from build123d import *

# Parameters (mm, degrees)
EXTRUDE_1_DEPTH      = 2
EXTRUDE_2_DEPTH      = 29
EXTRUDE_2_DEPTH_BACK = 2
CUT_EXTRUDE_5_REACH  = 63.117
SKETCH_3_R           = 0.75
SKETCH_3_W           = 9
SKETCH_3_H           = 20.1
CUT_EXTRUDE_7_REACH  = 63.924
SKETCH_12_R          = 0.75
SKETCH_12_W          = 9
SKETCH_12_H          = 20.1
CUT_EXTRUDE_8_REACH  = 75.269
SKETCH_13_R          = 1
SKETCH_13_W          = 16
SKETCH_13_H          = 40.897450577
EXTRUDE_START        = 15
SKETCH_15_R          = 2
SKETCH_15_R_2        = 1
EXTRUDE_9_DEPTH      = 15
CUT_EXTRUDE_9_REACH  = 63.508
SKETCH_16_W          = 5
SKETCH_16_H          = 20
EXTRUDE_10_DEPTH     = 24.1
EXTRUDE_11_DEPTH     = 1.5
CUT_EXTRUDE_10_REACH = 75.269
SKETCH_20_W          = 30
SKETCH_20_H          = 1.5
EXTRUDE_12_DEPTH     = 15
SKETCH_21_W          = 16
SKETCH_21_H          = 2
EXTRUDE_13_DEPTH     = 2
SKETCH_22_W          = 1
SKETCH_22_H          = 8
SKETCH_22_W_2        = 1.757464375
SKETCH_22_H_2        = 1.5298575
EXTRUDE_14_DEPTH     = 13
CUT_EXTRUDE_11_REACH = 64.018
SKETCH_23_W          = 12.5
SKETCH_23_H          = 12.2


with BuildPart() as part:
    # 草圖1 → 填料-伸長1 (new body)
    with BuildSketch(Plane.XY):
        Polygon((-15, 0), (15, 0), (17.19885826, 0), (20.767570176, -12.346175865), (15, -14), (15, -64), (-15, -64), (-15, -14), (-20.767570176, -12.346175865), (-17.227361215, 0), align=None)
    extrude(amount=EXTRUDE_1_DEPTH)

    # 草圖2 → 填料-伸長2 (add, two sides: drawn at the far end of the back side and taken through both)
    with BuildSketch(Plane.XY.offset(2).offset(-EXTRUDE_2_DEPTH_BACK)):
        Polygon((-19.940658108, -9.462390777), (19.934511943, -9.464160254), (20.767570176, -12.346175865), (11.154953216, -15.102549423), (-11.154953216, -15.102549423), (-20.767570176, -12.346175865), align=None)
    extrude(amount=EXTRUDE_2_DEPTH + EXTRUDE_2_DEPTH_BACK)

    # 草圖3 → 除料-伸長5 (cut, up to next)
    with BuildSketch(Plane(origin=(3.55693642, -17.281245681, 0), x_dir=(0.9612616959383193, 0.2756373558169973, 0), z_dir=(-0.2756373558169973, 0.9612616959383194, 0)), mode=Mode.PRIVATE) as cut_extrude_5_sk1:
        with Locations((13.397816779, -5.2)):
            Circle(SKETCH_3_R)
    cut_extrude_5_tool1 = extrude(cut_extrude_5_sk1.sketch, amount=CUT_EXTRUDE_5_REACH, mode=Mode.PRIVATE) & part.part
    # 草圖3 → 除料-伸長5 (cut, up to next)
    with BuildSketch(Plane(origin=(3.55693642, -17.281245681, 0), x_dir=(0.9612616959383193, 0.2756373558169973, 0), z_dir=(-0.2756373558169973, 0.9612616959383194, 0)), mode=Mode.PRIVATE) as cut_extrude_5_sk2:
        with Locations((13.397816779, -28.7)):
            Circle(SKETCH_3_R)
    cut_extrude_5_tool2 = extrude(cut_extrude_5_sk2.sketch, amount=CUT_EXTRUDE_5_REACH, mode=Mode.PRIVATE) & part.part
    # 草圖3 → 除料-伸長5 (cut, up to next)
    with BuildSketch(Plane(origin=(3.55693642, -17.281245681, 0), x_dir=(0.9612616959383193, 0.2756373558169973, 0), z_dir=(-0.2756373558169973, 0.9612616959383194, 0)), mode=Mode.PRIVATE) as cut_extrude_5_sk3:
        with Locations((13.397816779, -16.95)):
            Rectangle(SKETCH_3_W, SKETCH_3_H)
    cut_extrude_5_tool3 = extrude(cut_extrude_5_sk3.sketch, amount=CUT_EXTRUDE_5_REACH, mode=Mode.PRIVATE) & part.part
    add(cut_extrude_5_tool1.solids().sort_by_distance((16.435744, -13.588307, 5.2))[0], mode=Mode.SUBTRACT)
    add(cut_extrude_5_tool2.solids().sort_by_distance((16.435744, -13.588307, 28.7))[0], mode=Mode.SUBTRACT)
    add(cut_extrude_5_tool3.solids().sort_by_distance((16.435744, -13.588307, 16.95))[0], mode=Mode.SUBTRACT)

    # 除料-伸長7: up to this plane
    cut_extrude_7_end = Plane(origin=(-19.940658108, -9.462390777, 0), z_dir=(4.437541139610382e-05, 0.9999999990154116, 0))
    # 草圖12 → 除料-伸長7 (cut, up to the surface)
    with BuildSketch(Plane(origin=(-4.849074128, -16.910731155, 0), x_dir=(0.9612616959383179, -0.2756373558170027, 0), z_dir=(-0.2756373558170027, -0.9612616959383179, 0)), mode=Mode.PRIVATE) as cut_extrude_7_sk1:
        with Locations((-12.060002458, 28.7)):
            Circle(SKETCH_12_R)
    cut_extrude_7_tool1 = split(extrude(cut_extrude_7_sk1.sketch, amount=-CUT_EXTRUDE_7_REACH, mode=Mode.PRIVATE), bisect_by=cut_extrude_7_end, keep=Keep.BOTH, mode=Mode.PRIVATE)
    add(cut_extrude_7_tool1.solids().sort_by_distance((-16.441893, -13.586544, 28.7))[0], mode=Mode.SUBTRACT)
    # 草圖12 → 除料-伸長7 (cut, up to the surface)
    with BuildSketch(Plane(origin=(-4.849074128, -16.910731155, 0), x_dir=(0.9612616959383179, -0.2756373558170027, 0), z_dir=(-0.2756373558170027, -0.9612616959383179, 0)), mode=Mode.PRIVATE) as cut_extrude_7_sk2:
        with Locations((-12.060002458, 5.2)):
            Circle(SKETCH_12_R)
    cut_extrude_7_tool2 = split(extrude(cut_extrude_7_sk2.sketch, amount=-CUT_EXTRUDE_7_REACH, mode=Mode.PRIVATE), bisect_by=cut_extrude_7_end, keep=Keep.BOTH, mode=Mode.PRIVATE)
    add(cut_extrude_7_tool2.solids().sort_by_distance((-16.441893, -13.586544, 5.2))[0], mode=Mode.SUBTRACT)
    # 草圖12 → 除料-伸長7 (cut, up to the surface)
    with BuildSketch(Plane(origin=(-4.849074128, -16.910731155, 0), x_dir=(0.9612616959383179, -0.2756373558170027, 0), z_dir=(-0.2756373558170027, -0.9612616959383179, 0)), mode=Mode.PRIVATE) as cut_extrude_7_sk3:
        with Locations((-12.060002458, 16.95)):
            Rectangle(SKETCH_12_W, SKETCH_12_H)
    cut_extrude_7_tool3 = split(extrude(cut_extrude_7_sk3.sketch, amount=-CUT_EXTRUDE_7_REACH, mode=Mode.PRIVATE), bisect_by=cut_extrude_7_end, keep=Keep.BOTH, mode=Mode.PRIVATE)
    add(cut_extrude_7_tool3.solids().sort_by_distance((-16.441893, -13.586544, 16.95))[0], mode=Mode.SUBTRACT)

    # 草圖13 → 除料-伸長8 (cut, up to next)
    with BuildSketch(Plane.XY.offset(2), mode=Mode.PRIVATE) as cut_extrude_8_sk1:
        with Locations((-13, -34)):
            Circle(SKETCH_13_R)
    cut_extrude_8_tool1 = extrude(cut_extrude_8_sk1.sketch, amount=-CUT_EXTRUDE_8_REACH, mode=Mode.PRIVATE) & part.part
    # 草圖13 → 除料-伸長8 (cut, up to next)
    with BuildSketch(Plane.XY.offset(2), mode=Mode.PRIVATE) as cut_extrude_8_sk2:
        with Locations((13, -34)):
            Circle(SKETCH_13_R)
    cut_extrude_8_tool2 = extrude(cut_extrude_8_sk2.sketch, amount=-CUT_EXTRUDE_8_REACH, mode=Mode.PRIVATE) & part.part
    # 草圖13 → 除料-伸長8 (cut, up to next)
    with BuildSketch(Plane.XY.offset(2), mode=Mode.PRIVATE) as cut_extrude_8_sk3:
        with Locations((-13, -61.5)):
            Circle(SKETCH_13_R)
    cut_extrude_8_tool3 = extrude(cut_extrude_8_sk3.sketch, amount=-CUT_EXTRUDE_8_REACH, mode=Mode.PRIVATE) & part.part
    # 草圖13 → 除料-伸長8 (cut, up to next)
    with BuildSketch(Plane.XY.offset(2), mode=Mode.PRIVATE) as cut_extrude_8_sk4:
        with Locations((13, -61.5)):
            Circle(SKETCH_13_R)
    cut_extrude_8_tool4 = extrude(cut_extrude_8_sk4.sketch, amount=-CUT_EXTRUDE_8_REACH, mode=Mode.PRIVATE) & part.part
    # 草圖13 → 除料-伸長8 (cut, up to next)
    with BuildSketch(Plane.XY.offset(2), mode=Mode.PRIVATE) as cut_extrude_8_sk5:
        with Locations((0, -40.551274712)):
            Rectangle(SKETCH_13_W, SKETCH_13_H)
    cut_extrude_8_tool5 = extrude(cut_extrude_8_sk5.sketch, amount=-CUT_EXTRUDE_8_REACH, mode=Mode.PRIVATE) & part.part
    add(cut_extrude_8_tool1.solids().sort_by_distance((-13, -34, 2))[0], mode=Mode.SUBTRACT)
    add(cut_extrude_8_tool2.solids().sort_by_distance((13, -34, 2))[0], mode=Mode.SUBTRACT)
    add(cut_extrude_8_tool3.solids().sort_by_distance((-13, -61.5, 2))[0], mode=Mode.SUBTRACT)
    add(cut_extrude_8_tool4.solids().sort_by_distance((13, -61.5, 2))[0], mode=Mode.SUBTRACT)
    add(cut_extrude_8_tool5.solids().sort_by_distance((0, -40.551275, 2))[0], mode=Mode.SUBTRACT)

    # 草圖15 → 填料-伸長9 (add)
    # profile 1 of 4: a face of its own
    with BuildSketch(Plane.XY.offset(2).offset(EXTRUDE_START)):
        with Locations(Location((-13, -34, 0), (0, 0, 180))):
            Circle(SKETCH_15_R)
        with Locations((-13, -34)):
            Circle(SKETCH_15_R_2, mode=Mode.SUBTRACT)
    # profile 2 of 4: a face of its own
    with BuildSketch(Plane.XY.offset(2).offset(EXTRUDE_START)):
        with Locations((13, -34)):
            Circle(SKETCH_15_R)
        with Locations((13, -34)):
            Circle(SKETCH_15_R_2, mode=Mode.SUBTRACT)
    # profile 3 of 4: a face of its own
    with BuildSketch(Plane.XY.offset(2).offset(EXTRUDE_START)):
        with Locations((13, -61.5)):
            Circle(SKETCH_15_R)
        with Locations((13, -61.5)):
            Circle(SKETCH_15_R_2, mode=Mode.SUBTRACT)
    # profile 4 of 4: a face of its own
    with BuildSketch(Plane.XY.offset(2).offset(EXTRUDE_START)):
        with Locations(Location((-13, -61.5, 0), (0, 0, 180))):
            Circle(SKETCH_15_R)
        with Locations((-13, -61.5)):
            Circle(SKETCH_15_R_2, mode=Mode.SUBTRACT)
    extrude(amount=-EXTRUDE_9_DEPTH)

    # 草圖16 → 除料-伸長9 (cut, up to next)
    with BuildSketch(Plane.XZ.offset(15.102549423), mode=Mode.PRIVATE) as cut_extrude_9_sk1:
        with Locations((-4, 17)):
            Rectangle(SKETCH_16_W, SKETCH_16_H)
    cut_extrude_9_tool1 = extrude(cut_extrude_9_sk1.sketch, amount=-CUT_EXTRUDE_9_REACH, mode=Mode.PRIVATE) & part.part
    # 草圖16 → 除料-伸長9 (cut, up to next)
    with BuildSketch(Plane.XZ.offset(15.102549423), mode=Mode.PRIVATE) as cut_extrude_9_sk2:
        with Locations((4, 17)):
            Rectangle(SKETCH_16_W, SKETCH_16_H)
    cut_extrude_9_tool2 = extrude(cut_extrude_9_sk2.sketch, amount=-CUT_EXTRUDE_9_REACH, mode=Mode.PRIVATE) & part.part
    add(cut_extrude_9_tool1.solids().sort_by_distance((-4, -15.102549, 17))[0], mode=Mode.SUBTRACT)
    add(cut_extrude_9_tool2.solids().sort_by_distance((4, -15.102549, 17))[0], mode=Mode.SUBTRACT)

    # 草圖17 → 填料-伸長10 (add)
    with BuildSketch(Plane.XY.offset(31)):
        Polygon((-19.940658108, -9.462390777), (-20.767570176, -12.346175865), (-20.213148693, -12.505153667), (-19.340658109, -9.462417403), align=None)
        Polygon((19.334511943, -9.464133629), (19.934511943, -9.464160254), (20.767570176, -12.346175865), (20.207014757, -12.506912545), align=None)
    extrude(amount=-EXTRUDE_10_DEPTH)

    # 草圖18 → 填料-伸長11 (add)
    with BuildSketch(Plane(origin=(0, 0, 0), x_dir=(-1, 0, 0), z_dir=(0, 0, -1))):
        Polygon((-20.767570176, -12.346175865), (-15, -22), (-15, -14), align=None)
        Polygon((20.767570176, -12.346175865), (15, -14), (15, -22), align=None)
    extrude(amount=-EXTRUDE_11_DEPTH)

    # 草圖19 → 除料-伸長10 (cut, up to next)
    with BuildSketch(Plane.XY.offset(2), mode=Mode.PRIVATE) as cut_extrude_10_sk1:
        Polygon((-19.940658108, -9.462390777), (19.934511943, -9.464160254), (19.934511943, 2.341545169), (-19.940658108, 2.341545169), align=None)
    cut_extrude_10_tool1 = extrude(cut_extrude_10_sk1.sketch, amount=-CUT_EXTRUDE_10_REACH, mode=Mode.PRIVATE) & part.part
    add(cut_extrude_10_tool1.solids().sort_by_distance((-0.002575, -3.560865, 2))[0], mode=Mode.SUBTRACT)

    # 草圖20 → 填料-伸長12 (add)
    with BuildSketch(Plane(origin=(0, 0, 0), x_dir=(-1, 0, 0), z_dir=(0, 0, -1))):
        with Locations((0, -58.25)):
            Rectangle(SKETCH_20_W, SKETCH_20_H)
        with Locations((0, -41.25)):
            Rectangle(SKETCH_20_W, SKETCH_20_H)
    extrude(amount=-EXTRUDE_12_DEPTH)

    # 草圖21 → 填料-伸長13 (add)
    with BuildSketch(Plane(origin=(0, 0, 0), x_dir=(-1, 0, 0), z_dir=(0, 0, -1))):
        with Locations((0, -49.5)):
            Rectangle(SKETCH_21_W, SKETCH_21_H)
    extrude(amount=-EXTRUDE_13_DEPTH)

    # 草圖22 → 填料-伸長14 (add)
    with BuildSketch(Plane.XY.offset(15)):
        with Locations((14.5, -38)):
            Rectangle(SKETCH_22_W, SKETCH_22_H)
        with Locations((-14.5, -38)):
            Rectangle(SKETCH_22_W, SKETCH_22_H)
        with Locations((14.121267813, -59.76492875)):
            Rectangle(SKETCH_22_W_2, SKETCH_22_H_2)
        with Locations((-14.121267813, -59.76492875)):
            Rectangle(SKETCH_22_W_2, SKETCH_22_H_2)
    extrude(amount=-EXTRUDE_14_DEPTH)

    # 除料-伸長11: up to this face of the body (flat: up to its plane)
    cut_extrude_11_end = Plane(part.part.faces().sort_by_distance((0, -40.5, 7.893939394))[0])
    # 草圖23 → 除料-伸長11 (cut, up to the picked face)
    with BuildSketch(Plane.XZ.offset(59), mode=Mode.PRIVATE) as cut_extrude_11_sk1:
        with Locations((0, 8.1)):
            Rectangle(SKETCH_23_W, SKETCH_23_H)
    cut_extrude_11_tool1 = split(extrude(cut_extrude_11_sk1.sketch, amount=-CUT_EXTRUDE_11_REACH, mode=Mode.PRIVATE), bisect_by=cut_extrude_11_end, keep=Keep.BOTH, mode=Mode.PRIVATE)
    add(cut_extrude_11_tool1.solids().sort_by(Axis((0, -59, 8.1), (0, 1, 0)))[0], mode=Mode.SUBTRACT)


solid = part.part
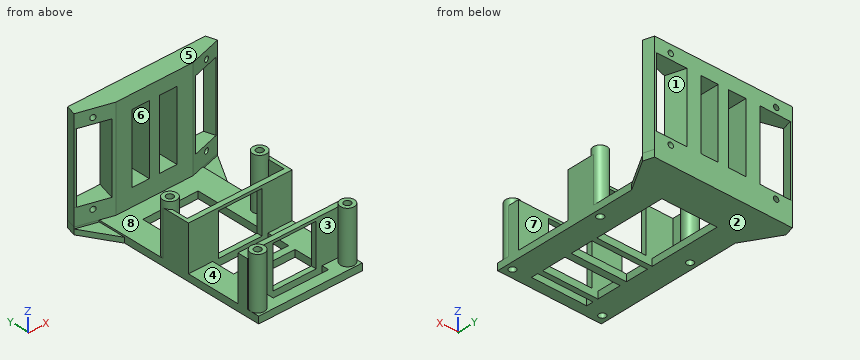
Can you work these out from the model? Positions are in its coordinate system, mm. Face numbers are marked on the shaded views. A direction names the side the tool comes from. Coordinates: 2 decimals unless noted, no trailing zeros. Write each loop counter-clockwise with the first axis right and the second up, starting at its lowest first coordinate (ties: lowest second). Pieces come first, ordered by that corner, then holes. Notation, with made-up numbers: (-13, -21.75) -> (44, -21.75) arc R19 ccw to (44, -1.75) -> close; hole circle Ø11 at (70.5, 33.25). An arc over 180 degrees is marked (long way). Answer as CSV lines item,"result".
1) If we section it at C-C on z = 12.5: Count the separate pieces of the cut face and the enclosed holes in it, then the cut area to 3 significant figures.
Check result:
separate pieces,"9"
enclosed holes,"4"
area,"179 mm²"
2) Will these pins go through, and if not, where does the flat tip stop? P1, Ø2.5, axis at x = -13, y = -61.5, coming from the +Z side; P2, Ø1, axis at y = -53.5, z = 1, coming from the -X side; P3, Ø12.5, axis at x = -5, y = -46, coming from the +Z side; P4, Ø1, axis at x = -5.5, y = -52, coming from the +Z side.
Check result:
P1,"z = 17"
P2,"x = -15"
P3,"z = 15"
P4,"through"
3) If we section it at D-D on x = -9: Please give me the cut outline in (y, z).
Check result:
outline,"(-64, 0) -> (-9.46, 0) -> (-9.46, 31) -> (-15.1, 31) -> (-15.1, 2) -> (-40.5, 2) -> (-40.5, 15) -> (-42, 15) -> (-42, 2) -> (-57.5, 2) -> (-57.5, 15) -> (-59, 15) -> (-59, 2) -> (-64, 2) -> close"
4) If we section it at B-B on y = -29.5: Please give me the cut outline in (x, z).
Check result:
outline,"(-15, 0) -> (-8, 0) -> (-8, 2) -> (-15, 2) -> close; (8, 0) -> (15, 0) -> (15, 2) -> (8, 2) -> close"
5) On a 3-axis mill with a long thin cutter (end or side, diameter ignored), from which of +Z, -Z, +X, -X, +Y, -Y can I reach the whole of each face in a straight line? I mean the marked faces 1, 2, 3, 4 and 5. Say none if no direction works.
Check result:
face 1,"+Y"
face 2,"-Z, +X, -X, +Y, -Y"
face 3,"+Z"
face 4,"+Z, +X, -X"
face 5,"+Z, +X, -X, +Y, -Y"
6) If we mould it in two halves opening along Z, with no side actions, what happens to the marked faces 6, 7 and 8? For each: +Z half, -Z half, draft (parallel to the pull), parting line (faces both ways), or undercut.
Check result:
face 6,"undercut"
face 7,"draft"
face 8,"+Z half"
7) If we section it at A-A on z = 23.5: Please give me the cut outline in (x, y).
Check result:
outline,"(-20.77, -12.35) -> (-20.21, -12.51) -> (-19.34, -9.46) -> (-19.94, -9.46) -> close; (-12.12, -14.83) -> (-11.15, -15.1) -> (-6.5, -15.1) -> (-6.5, -9.46) -> (-10.58, -9.46) -> close; (-1.5, -15.1) -> (1.5, -15.1) -> (1.5, -9.46) -> (-1.5, -9.46) -> close; (6.5, -15.1) -> (11.15, -15.1) -> (12.11, -14.83) -> (10.57, -9.46) -> (6.5, -9.46) -> close; (19.33, -9.46) -> (20.21, -12.51) -> (20.77, -12.35) -> (19.93, -9.46) -> close"
8) If I drill on line 1 (Y direction, x = -13, z = 10.75); line 2 (Z direction, x = -4, y = -12.5); line 3 (X direction, y = -13, z = 16), over which ranges is the centre line in solid material (lowest first)? Write a range as from..to.
Check result:
line 1,"-63.5..-62.5, -60.5..-59.5, -59..-57.5, -42..-40.5, -36..-35, -33..-32"
line 2,"0..7, 27..31"
line 3,"-11.59..-6.5, -1.5..1.5, 6.5..11.59"
